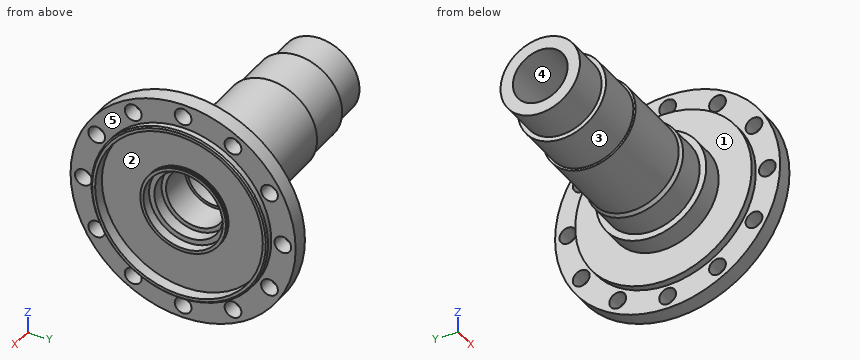
```python
from build123d import *

# Parameters (mm, degrees)
SKETCH_3_W           = 2
SKETCH_3_H           = 46.5
SKETCH_5_W           = 2
SKETCH_5_H           = 46.5
SKETCH_6_R           = 9.5
CUT_EXTRUDE_1_DEPTH  = 328.171973127
SKETCH_7_R           = 9.5
CUT_EXTRUDE_2_DEPTH  = 328.171973127
SKETCH_8_R           = 9.5
CUT_EXTRUDE_3_DEPTH  = 328.171973127
SKETCH_9_R           = 9.5
CUT_EXTRUDE_4_DEPTH  = 328.171973127
SKETCH_10_R          = 9.5
CUT_EXTRUDE_5_DEPTH  = 328.171973127
SKETCH_11_R          = 9.5
CUT_EXTRUDE_6_DEPTH  = 328.171973127
SKETCH_12_R          = 9.5
CUT_EXTRUDE_7_DEPTH  = 328.171973127
SKETCH_13_R          = 9.5
CUT_EXTRUDE_8_DEPTH  = 328.171973127
SKETCH_14_R          = 9.5
CUT_EXTRUDE_9_DEPTH  = 328.171973127
SKETCH_15_R          = 9.5
CUT_EXTRUDE_10_DEPTH = 328.171973127
SKETCH_16_R          = 9.5
CUT_EXTRUDE_11_DEPTH = 328.171973127
SKETCH_17_R          = 9.5
CUT_EXTRUDE_12_DEPTH = 328.171973127


with BuildPart() as part:
    # Эскиз1 → Повернуть1 (revolve)
    with BuildSketch(Plane.XY, mode=Mode.PRIVATE) as revolve_1_sk:
        Polygon((0, 0), (273, 0), (273, 98.4), (271.4, 100), (265, 100), (265, 127.5), (247, 127.5), (247, 100), (239, 100), (239, 62.5), (215, 62.5), (215, 55), (183, 55), (178.669872981, 52.5), (95, 52.5), (95, 50), (42, 50), (42, 45), (0, 45), align=None)
    revolve(revolve_1_sk.sketch.rotate(Axis((0, 0, 0), (1, 0, 0)), 90), axis=Axis((0, 0, 0), (1, 0, 0)))

    # Эскиз2 → Вырез-Повернуть1 (revolve, cut)
    with BuildSketch(Plane.XY, mode=Mode.PRIVATE) as cut_revolve_1_sk:
        Polygon((0, 0), (273, 0), (273, 95), (265, 95), (265, 45), (254, 45), (254, 39), (240, 39), (240, 34), (203.5, 34), (203.5, 31), (0, 31), align=None)
    revolve(cut_revolve_1_sk.sketch.rotate(Axis((0, 0, 0), (1, 0, 0)), 90), axis=Axis((0, 0, 0), (1, 0, 0)), mode=Mode.SUBTRACT)

    # Эскиз3 → Rear_recess_left (revolve, cut)
    with BuildSketch(Plane.XY, mode=Mode.PRIVATE) as rear_recess_left_sk:
        with Locations((261, 71.75)):
            Rectangle(SKETCH_3_W, SKETCH_3_H)
    revolve(rear_recess_left_sk.sketch.rotate(Axis((0, 0, 0), (1, 0, 0)), 90), axis=Axis((0, 0, 0), (1, 0, 0)), mode=Mode.SUBTRACT)

    # Эскиз4 → Collar_groove_nominal (revolve, cut)
    with BuildSketch(Plane.XY, mode=Mode.PRIVATE) as collar_groove_nominal_sk:
        with BuildLine():
            Line((263, 48), (263, 95))
            Line((263, 95), (262, 95))
            Line((262, 95), (262, 48))
            ThreePointArc((262, 48), (262.146446609, 47.646446609), (262.5, 47.5))
            ThreePointArc((262.5, 47.5), (262.853553391, 47.646446609), (263, 48))
        make_face()
    revolve(collar_groove_nominal_sk.sketch.rotate(Axis((0, 0, 0), (1, 0, 0)), 90), axis=Axis((0, 0, 0), (1, 0, 0)), mode=Mode.SUBTRACT)

    # Эскиз5 → Rear_recess_lip (revolve, cut)
    with BuildSketch(Plane.XY, mode=Mode.PRIVATE) as rear_recess_lip_sk:
        with Locations((264, 71.75)):
            Rectangle(SKETCH_5_W, SKETCH_5_H)
    revolve(rear_recess_lip_sk.sketch.rotate(Axis((0, 0, 0), (1, 0, 0)), 90), axis=Axis((0, 0, 0), (1, 0, 0)), mode=Mode.SUBTRACT)

    # Эскиз6 → Вырез-Вытянуть1 (cut, through all)
    with BuildSketch(Plane(origin=(0, 0, 0), x_dir=(0, 0, -1), z_dir=(1, 0, 0))):
        with Locations(Location((0, 113, 0), (0, 0, 180))):
            Circle(SKETCH_6_R)
    extrude(amount=CUT_EXTRUDE_1_DEPTH, mode=Mode.SUBTRACT)

    # Эскиз7 → Вырез-Вытянуть2 (cut, through all)
    with BuildSketch(Plane(origin=(0, 0, 0), x_dir=(0, 0, -1), z_dir=(1, 0, 0))):
        with Locations(Location((-56.5, 97.860870628, 0), (0, 0, 180))):
            Circle(SKETCH_7_R)
    extrude(amount=CUT_EXTRUDE_2_DEPTH, mode=Mode.SUBTRACT)

    # Эскиз8 → Вырез-Вытянуть3 (cut, through all)
    with BuildSketch(Plane(origin=(0, 0, 0), x_dir=(0, 0, -1), z_dir=(1, 0, 0))):
        with Locations(Location((-97.860870628, 56.5, 0), (0, 0, 180))):
            Circle(SKETCH_8_R)
    extrude(amount=CUT_EXTRUDE_3_DEPTH, mode=Mode.SUBTRACT)

    # Эскиз9 → Вырез-Вытянуть4 (cut, through all)
    with BuildSketch(Plane(origin=(0, 0, 0), x_dir=(0, 0, -1), z_dir=(1, 0, 0))):
        with Locations(Location((-113, 0, 0), (0, 0, 180))):
            Circle(SKETCH_9_R)
    extrude(amount=CUT_EXTRUDE_4_DEPTH, mode=Mode.SUBTRACT)

    # Эскиз10 → Вырез-Вытянуть5 (cut, through all)
    with BuildSketch(Plane(origin=(0, 0, 0), x_dir=(0, 0, -1), z_dir=(1, 0, 0))):
        with Locations(Location((-97.860870628, -56.5, 0), (0, 0, 180))):
            Circle(SKETCH_10_R)
    extrude(amount=CUT_EXTRUDE_5_DEPTH, mode=Mode.SUBTRACT)

    # Эскиз11 → Вырез-Вытянуть6 (cut, through all)
    with BuildSketch(Plane(origin=(0, 0, 0), x_dir=(0, 0, -1), z_dir=(1, 0, 0))):
        with Locations(Location((-56.5, -97.860870628, 0), (0, 0, 180))):
            Circle(SKETCH_11_R)
    extrude(amount=CUT_EXTRUDE_6_DEPTH, mode=Mode.SUBTRACT)

    # Эскиз12 → Вырез-Вытянуть7 (cut, through all)
    with BuildSketch(Plane(origin=(0, 0, 0), x_dir=(0, 0, -1), z_dir=(1, 0, 0))):
        with Locations(Location((0, -113, 0), (0, 0, 180))):
            Circle(SKETCH_12_R)
    extrude(amount=CUT_EXTRUDE_7_DEPTH, mode=Mode.SUBTRACT)

    # Эскиз13 → Вырез-Вытянуть8 (cut, through all)
    with BuildSketch(Plane(origin=(0, 0, 0), x_dir=(0, 0, -1), z_dir=(1, 0, 0))):
        with Locations(Location((56.5, -97.860870628, 0), (0, 0, 180))):
            Circle(SKETCH_13_R)
    extrude(amount=CUT_EXTRUDE_8_DEPTH, mode=Mode.SUBTRACT)

    # Эскиз14 → Вырез-Вытянуть9 (cut, through all)
    with BuildSketch(Plane(origin=(0, 0, 0), x_dir=(0, 0, -1), z_dir=(1, 0, 0))):
        with Locations(Location((97.860870628, -56.5, 0), (0, 0, 180))):
            Circle(SKETCH_14_R)
    extrude(amount=CUT_EXTRUDE_9_DEPTH, mode=Mode.SUBTRACT)

    # Эскиз15 → Вырез-Вытянуть10 (cut, through all)
    with BuildSketch(Plane(origin=(0, 0, 0), x_dir=(0, 0, -1), z_dir=(1, 0, 0))):
        with Locations(Location((113, 0, 0), (0, 0, 180))):
            Circle(SKETCH_15_R)
    extrude(amount=CUT_EXTRUDE_10_DEPTH, mode=Mode.SUBTRACT)

    # Эскиз16 → Вырез-Вытянуть11 (cut, through all)
    with BuildSketch(Plane(origin=(0, 0, 0), x_dir=(0, 0, -1), z_dir=(1, 0, 0))):
        with Locations(Location((97.860870628, 56.5, 0), (0, 0, 180))):
            Circle(SKETCH_16_R)
    extrude(amount=CUT_EXTRUDE_11_DEPTH, mode=Mode.SUBTRACT)

    # Эскиз17 → Вырез-Вытянуть12 (cut, through all)
    with BuildSketch(Plane(origin=(0, 0, 0), x_dir=(0, 0, -1), z_dir=(1, 0, 0))):
        with Locations(Location((56.5, 97.860870628, 0), (0, 0, 180))):
            Circle(SKETCH_17_R)
    extrude(amount=CUT_EXTRUDE_12_DEPTH, mode=Mode.SUBTRACT)


solid = part.part
```
CAD build for the part. Positions are in the model's coordinates, mm. Face numbers are marked on the shaded views. A direction names the side the tool comes from. Coordinates: 2 decimals unless noted, no trailing zeros. Write each loop counter-clockwise with the first axis right and the second up, starting at its lowest first coordinate (ties: lowest second). Pieces come first, ordered by that corner, then holes. Notation, with made-up numbers: (-34, 9.25) -> (-8, 9.25) arc R23 ccw to (-8, 40.25) -> close; hole circle Ø5 at (63, 66). An arc over 180 degrees is marked (long way). Use CSV: the item, a comma, the result in double quotes. Start each with the question number.
Item 1: Two-plate mould, pull along Y, no slides. Class the marked faces 3, 4 and 5: +Y half, -Y half, draft (parallel to the pull), parting line (faces both ways), or undercut.
Item 2: Band-saw the part on D-D, the plane x = 58. Write the cut outline in (y, z).
Item 3: Band-saw the part on A-A, the plane y = -113. Write the cut outline in (x, z).
Item 4: Tool access for the marked faces 1 and 2: list every direction of +Z, -Z, +X, -X, +Y, -Y with a clear straight run to the whole face (end or side of a thin tool).
Item 5: Drop flat-ended pins along their axis: P1, Ø17, axis at y = -97.86, z = 56.5, coming from the +X side; P2, Ø1, axis at y = 88.5, z = 86, coming from the -X side; P3, Ø4, axis at y = -65.5, z = 55.5, coming from the -X side; P4, Ø10, axis at x = 225, z = -40.5, coming from the -Y side. Give the stop position or say it passes through.
Item 6: Wall check: probe 1 along Y at (x, z) = (255, 0); probe 2 along Y at (x, z) = (56, 0); probe 3 along Y at (x, z) = (264.5, 0). Give the ranges that are in metal, low to high.
Item 7: Band-saw the part on C-C, the plane x = 132. Write the cut outline in (y, z), plus the area to 3 significant figures.
Response values:
1,face 3,"parting line"
1,face 4,"undercut"
1,face 5,"draft"
2,outline,"circle Ø100 at (0, 0); hole circle Ø62 at (0, 0)"
3,outline,"(247, -59.05) -> (265, -59.05) -> (265, -9.5) -> (247, -9.5) -> close; (247, 9.5) -> (265, 9.5) -> (265, 59.05) -> (247, 59.05) -> close"
4,face 1,"-X"
4,face 2,"+X"
5,P1,"passes through"
5,P2,"stops at x = 247"
5,P3,"stops at x = 239"
5,P4,"stops at y = -51.44"
6,probe 1,"y = -127.5 to -122.5, -103.5 to -45, 45 to 103.5, 122.5 to 127.5"
6,probe 2,"y = -50 to -31, 31 to 50"
6,probe 3,"y = -127.5 to -122.5, -103.5 to -95, -48.5 to -45, 45 to 48.5, 95 to 103.5, 122.5 to 127.5"
7,outline,"circle Ø105 at (0, 0); hole circle Ø62 at (0, 0)"
7,area,"5,640 mm2"
